Input: part model. Units: mm. Frame: model coordinates. A direction names the side the tool comes from. Round coordinates to 2 decimals unless told otherwise and drop trailing zeros. Loops run counter-clockwise (first coordinate to the right, second up) from the corner with the lowest first, then second, coordinate; pieces in that order, holes last. Notation, with made-up numbers: (3, -18) -> (31, -18) arc R14 cw to (31, 2) -> close; hole circle Ø6 at (74.5, 85). An arc over 180 degrees is marked (long way). Answer in a Markdown table with one row per item. Add a question column.
Q1. Section B-B, the plane y = 2.3. Output: boundary loops of the cut face in (x, z).
Q2. Pin query (flat end, axial travel): pin 1 (1.5 mm diameter, centred on y = 2, z = -3, fed in from +X); pin 2 (2 mm diameter, centred on x = 4.5, z = 4, fed in from +Y). Return the tip coordinate at first contact, or that it passes through.
Q3. Ray query, L1, parallel to X at y = 1.95, z = 0; L2, parallel to Y at x = -5.25, z = 3.75. Return the intervals inside material, ascending. Write a range as from..to.
Q4. Reachability of faces 1 (the face through (0, 0, -3)), 2 (the face through (-0.59, 2.12, 4.46)) from +Z, -Z, +X, -X, +Y, -Y: full face, straight path, thin tool, end or side. Return the list, or none.
Q5. Section C-C, the plane y = 1.5. Output: boundary loops of the cut face in (x, z), and give its area (3 significant figures).
Autodesk Inventor part; units mm, degrees
ref_plane "YZ Plane" through (0, 0, 0) normal (1, 0, 0) x (0, 1, 0)
ref_plane "XZ Plane" through (0, 0, 0) normal (0, 1, 0) x (-1, 0, 0)
ref_plane "XY Plane" through (0, 0, 0) normal (0, 0, 1) x (1, 0, 0)
sketch "Sketch1" plane through (0, 0, 0) normal (0, 1, 0) x (-1, 0, 0)
  circle A0 centre (0, 0) radius 2.8
  circle A1 centre (0, 0) radius 7.5
  dimension "d0" = 5.6
  dimension "d1" = 15
extrude "Extrusion1" add sketch "Sketch1" along normal blind 1.75
sketch "Sketch2" plane through (0, 1.75, 0) normal (0, 1, 0) x (1, 0, 0)
  circle A0 centre (0, 0) radius 4.5
  circle A1 centre (0, 0) radius 2.8
  dimension "d4" = 9
extrude "Extrusion2" add sketch "Sketch2" along normal blind 0.75
chamfer "Chamfer1" distance 1 angle 45 1 edges at (7.5, 1.75, 0)
properties part number "x carraige sliding spacer short" material "ABS Plastic"
Answer block:
| question | item | result |
|---|---|---|
| 1 | outline | circle Ø9 at (0, 0); hole circle Ø5.6 at (0, 0) |
| 2 | pin 1 | x = 6.39 |
| 2 | pin 2 | y = 1.75 |
| 3 | L1 | -4.5..-2.8, 2.8..4.5 |
| 3 | L2 | 0..1.75 |
| 4 | face 1 | +Z, -Z, +X, -X, -Y |
| 4 | face 2 | +Y |
| 5 | outline | circle Ø13.5 at (0, 0); hole circle Ø5.6 at (0, 0) |
| 5 | area | 119 mm^2 |
